The model under review builds one solid part; all positions refer to its coordinate system, in mm. Face numbers are marked on the shaded views. A direction names the side the tool comes from. Give positions to 0.01 mm unless a question says otherwise; leave off trailing zeros. Loops run counter-clockwise (first coordinate to the right, second up) from the corner with the lowest first, then second, coordinate; pieces in that order, holes last. Notation, with made-up numbers: (17.25, -24.5) - (44.25, -24.5) arc R22 cw to (44.25, -17.5) - close; hole circle Ø6 at (-1, 89.5). An arc over 180 degrees is marked (long way). Answer as a JSON object with one key per item and string values.
from build123d import *

# Parameters (mm, degrees)
F1_DEPTH = 75
F3_D     = 13
F3_DEPTH = 500
F4_R     = 15


with BuildPart() as f1:
    # F0 (on Right) → F1 (new body)
    with BuildSketch(Plane.YZ):
        with BuildLine():
            Line((-64, 134), (-64, 0))
            Line((-64, 0), (-60, 0))
            Line((-60, 0), (-60, 130))
            ThreePointArc((-60, 130), (-57.071068, 137.071068), (-50, 140))
            Line((-50, 140), (50, 140))
            ThreePointArc((50, 140), (57.071068, 137.071068), (60, 130))
            Line((60, 130), (60, 0))
            Line((60, 0), (64, 0))
            Line((64, 0), (64, 134))
            ThreePointArc((64, 134), (61.071068, 141.071068), (54, 144))
            Line((54, 144), (-54, 144))
            ThreePointArc((-54, 144), (-61.071068, 141.071068), (-64, 134))
        make_face()
    extrude(amount=F1_DEPTH)

    # F3
    with Locations(Plane.XZ.offset(64)):
        with Locations((37.5, 19)):
            Hole(F3_D / 2, depth=F3_DEPTH)

    # F4
    f4_edges = [f1.edges().sort_by_distance(p)[0] for p in [
        (0, -62, 0),
        (75, -62, 0),
        (75, 62, 0),
        (0, 62, 0),
    ]]
    fillet(f4_edges, radius=F4_R)


solid = f1.part
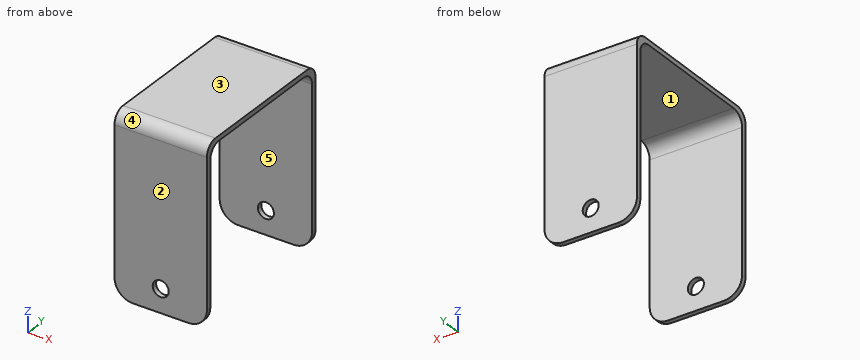
Q1. Consider section D-D, the plane y = 19. State the section outline as (x, z) points, plus the area to 3 significant figures.
Results:
{"outline": "(0, 140) - (75, 140) - (75, 144) - (0, 144) - close", "area": "300 mm^2"}
Q2. The part is to be moulded in two halves that separate along Y. For the marked faces 1, 2 and 3, say which applies: +Y half, -Y half, draft (parallel to the pull), parting line (faces both ways), or undercut.
Results:
{"face 1": "undercut", "face 2": "-Y half", "face 3": "draft"}
Q3. Consider section A-A, the plane x = 37.5. State the section outline as (y, z) points.
Results:
{"outline": "(-64, 0) - (-60, 0) - (-60, 12.5) - (-64, 12.5) - close; (-64, 25.5) - (-60, 25.5) - (-60, 130) arc R10 cw to (-50, 140) - (50, 140) arc R10 cw to (60, 130) - (60, 25.5) - (64, 25.5) - (64, 134) arc R10 ccw to (54, 144) - (-54, 144) arc R10 ccw to (-64, 134) - close; (60, 0) - (64, 0) - (64, 12.5) - (60, 12.5) - close"}
Q4. Consider section C-C, the plane z = 19. State the section outline as (x, y) points, plus the area to 3 significant figures.
Results:
{"outline": "(0, -64) - (31, -64) - (31, -60) - (0, -60) - close; (0, 60) - (31, 60) - (31, 64) - (0, 64) - close; (44, -64) - (75, -64) - (75, -60) - (44, -60) - close; (44, 60) - (75, 60) - (75, 64) - (44, 64) - close", "area": "496 mm^2"}
Q5. For the marked faces 4 and 5, list the 3-axis set-ups (+Z, -Z, +X, -X, +Y, -Y) from which the entire face can be reached by the end or side of a thin tool; tool diameter is ignored.
Results:
{"face 4": "+Z, +X, -X, -Y", "face 5": "-Z, +X, -X"}
Q6. Clearance check with a flat-ended pin moving along its axis: pin 1 Ø6 at (x, y) = (25, -20) entering from -Z. State where the tip first meets the part, or that it passes through.
Results:
{"pin 1": "stops at z = 140"}
Q7. To check wall thickness, follow probe 1 along Y at (x, z) = (63.5, 104); probe 2 along Z at (x, y) = (49, 7.5); probe 3 along Z at (x, y) = (37, 61). State the ranges of each line that lie inside material, in increasing order. Write a range as [from, to].
Results:
{"probe 1": "y = [-64, -60], [60, 64]", "probe 2": "z = [140, 144]", "probe 3": "z = [0, 12.52], [25.48, 141.14]"}
Q8. Consider section B-B, the plane z = 127. State the section outline as (x, y) points.
Results:
{"outline": "(0, -64) - (75, -64) - (75, -60) - (0, -60) - close; (0, 60) - (75, 60) - (75, 64) - (0, 64) - close"}
